Verification items for the finished model (mm, model axes). A direction names the side the tool comes from. Round coordinates to 2 decimals unless told otherwise and drop trailing zeros. Loops run counter-clockwise (first coordinate to the right, second up) from the corner with the lowest first, then second, coordinate; pieces in that order, holes last. Notation, with made-up numbers: (36, -14) -> (60, -14) arc R28 cw to (60, 10) -> close; hole circle Ø8 at (60, -25). An arc over 180 degrees is marked (long way). Use CSV: the item, a comma, the result in double quotes. Start each with the question number.
```python
from build123d import *

# Parameters (mm, degrees)
SALIENTE_EXTRUIR1_DEPTH    = 75
CORTAR_EXTRUIR1_REACH      = 405.099
CROQUIS2_R                 = 45
CORTAR_EXTRUIR2_REACH      = 397.531
CORTAR_EXTRUIR2_END_RADIUS = 165


with BuildPart() as part:
    # Croquis1 → Saliente-Extruir1 (new, symmetric)
    with BuildSketch(Plane.XY):
        with BuildLine():
            Line((-10, 250), (0, 250))
            Line((0, 250), (0, 0))
            Line((0, 0), (-234.378862456, 0))
            ThreePointArc((-234.378862456, 0), (-306.168920604, 118.546607009), (-262.269991763, 250))
            Line((-262.269991763, 250), (-248.111243039, 250))
            ThreePointArc((-248.111243039, 250), (-296.806166022, 125.992691614), (-231.272178278, 10))
            Line((-231.272178278, 10), (-10, 10))
            Line((-10, 10), (-10, 250))
        make_face()
    extrude(amount=SALIENTE_EXTRUIR1_DEPTH, both=True)

    # Croquis2 → Cortar-Extruir1 (cut, up to next)
    with BuildSketch(Plane(origin=(0, 0, 0), x_dir=(0, 0, -1), z_dir=(1, 0, 0)), mode=Mode.PRIVATE) as cortar_extruir1_sk1:
        with Locations(Location((0, 136.841249694, 0), (0, 0, 90))):
            Circle(CROQUIS2_R)
    cortar_extruir1_tool1 = extrude(cortar_extruir1_sk1.sketch, amount=-CORTAR_EXTRUIR1_REACH, mode=Mode.PRIVATE) & part.part
    add(cortar_extruir1_tool1.solids().sort_by_distance((0, 136.84125, 0))[0], mode=Mode.SUBTRACT)

    # Cortar-Extruir2: up to this cylinder (the profile starts inside it)
    cortar_extruir2_end = Plane(origin=(-142.186281275, 136.841251, 0), z_dir=(0, 0, -1)) * Cylinder(CORTAR_EXTRUIR2_END_RADIUS, 1126.062, mode=Mode.PRIVATE)
    # Croquis3 → Cortar-Extruir2 (cut, up to the surface)
    with BuildSketch(Plane.ZY.offset(10), mode=Mode.PRIVATE) as cortar_extruir2_sk1:
        with BuildLine():
            Line((45, 185), (45, 65))
            ThreePointArc((45, 65), (0, 20), (-45, 65))
            Line((-45, 65), (-45, 185))
            ThreePointArc((-45, 185), (0, 230), (45, 185))
        make_face()
    cortar_extruir2_tool1 = extrude(cortar_extruir2_sk1.sketch, amount=CORTAR_EXTRUIR2_REACH, mode=Mode.PRIVATE) & cortar_extruir2_end
    add(cortar_extruir2_tool1.solids().sort_by_distance((-10, 125, 0))[0], mode=Mode.SUBTRACT)


solid = part.part
```
Q1. Depth check by flat-ended pin: pin 1 Ø10 at (y, z) = (168, -47.5) entering from -X; pin 2 Ø8 at (y, z) = (62, 46) entering from -X; pin 3 Ø12 at (y, z) = (89, 52) entering from -X. Enter the tip coordinate at first touch or a pass-through.
Q2. Cross-section at C-C (y = 48). Record the boundary of the cut face in (x, z).
Q3. Cross-section at A-A (z = 17). Record the boundary of the cut face in (x, y).
Q4. Thickness scan on L1, parallel to X at y = 93.5, z = -34.5; L2, parallel to X at y = 74.5, z = 51; L3, parallel to X at y = 149.5, z = 57. Record the ranges inside material, lowest first. Write a range as from..to.
Q5. Tool access check on faces 4 (the face through (-277.774, 229.733, 4.896)), 5 (the face through (-256.68, 20.344, 5.552)), 6 (the face through (-122, 10, 1)), 7 (the face through (-296.93, 127.92, 51.05)), 8 (the face through (-4.93, 91.885, 1.979)). Record the directions out of +Z, -Z, +X, -X, +Y, -Y that give a thin tool (end or side, any length) a straight path to the whole face; none if there is none.
Q6. Cross-section at B-B (y = 145.5). Record the boundary of the cut face in (x, z), and give its area (3 significant figures).
Q7. Cross-section at D-D (z = -62). Record the boundary of the cut face in (x, y), and give its area (3 significant figures).
Q8. Release check for a two-part mould opening along X. For faces 1 (the face through (-130, 5, 75)), 2 (the face through (-10, 102, 34)), 3 (the face through (-305.935, 116.558, -48.95)) record: +X half, -X half, draft (parallel to the pull), parting line (faces both ways), or undercut.
Answer list:
1,pin 1,"stops at x = -305.1"
1,pin 2,"stops at x = -291.2"
1,pin 3,"stops at x = -301.79"
2,outline,"(-281.23, -75) -> (-269.2, -75) -> (-269.2, -41.67) -> (-281.23, -41.67) -> close; (-281.23, 41.67) -> (-269.2, 41.67) -> (-269.2, 75) -> (-281.23, 75) -> close; (-10, -75) -> (0, -75) -> (0, 75) -> (-10, 75) -> close"
3,outline,"(-280.59, 226.67) -> (-268.51, 226.67) arc R155 cw to (-248.11, 250) -> (-262.27, 250) arc R165 ccw to start; (-261.94, 23.33) arc R165 ccw to (-234.38, 0) -> (0, 0) -> (0, 95.18) -> (-10, 95.18) -> (-10, 10) -> (-231.27, 10) arc R155 cw to (-247.74, 23.33) -> close; (-10, 178.51) -> (0, 178.51) -> (0, 250) -> (-10, 250) -> close"
4,L1,"x = -10..0"
4,L2,"x = -294.96..-284.1, -10..0"
4,L3,"x = -306.7..-296.67, -10..0"
5,face 4,"-X, -Y"
5,face 5,"-X"
5,face 6,"+Z, -Z, +Y"
5,face 7,"+Z, -Z"
5,face 8,"+X, -X"
6,outline,"(-306.96, -75) -> (-296.94, -75) -> (-296.94, -45) -> (-306.96, -45) -> close; (-306.96, 45) -> (-296.94, 45) -> (-296.94, 75) -> (-306.96, 75) -> close; (-10, -75) -> (0, -75) -> (0, -44.16) -> (-10, -44.16) -> close; (-10, 44.16) -> (0, 44.16) -> (0, 75) -> (-10, 75) -> close"
6,area,"1,220 mm2"
7,outline,"(-262.27, 250) arc R165 ccw to (-234.38, 0) -> (0, 0) -> (0, 250) -> (-10, 250) -> (-10, 10) -> (-231.27, 10) arc R155 cw to (-248.11, 250) -> close"
7,area,"7,540 mm2"
8,face 1,"draft"
8,face 2,"undercut"
8,face 3,"-X half"
